The listing builds one solid part. Answer for the finished solid, in the listing's coordinates (mm). A direction names the side the tool comes from. Give positions to 0.01 mm unless a question says otherwise; leave off trailing zeros. Order: outer loops, then holes, each group sorted by start corner. A loop starts at its lowest first (then second) coordinate and runs counter-clockwise, first axis right, second up. Notation, with made-up numbers: (-8, -38.5) - (40, -38.5) arc R36 cw to (40, -3.5) - close; hole circle Ø11 at (58.25, -22.75). An arc over 180 degrees is marked (long way). Use a Markdown table: item, result. Add a question column.
1) Flat-ended cylindrical pins translate along their axes: pin 1 (10 mm diameter, centred on x = 62.5, y = 68, fed in from +Z); pin 2 (8 mm diameter, centred on y = 23, z = 55.5, fed in from -X); pin 3 (5 mm diameter, centred on x = 46.5, z = 36.5, fed in from -Y). Find the tip coordinate at first contact, or state that the pin passes through.
2) Find section B-B, the plane x = 10.5. Determine the outline of the cut face in (y, z), plus the area to 3 significant figures.
3) The mould has two halves that part along Z. Classify faces 1 (the face through (60.14, 45.69, 18.14)), 2 (the face through (112.2, 9.4, 97.8)), 3 (the face through (131.14, 46, 130)), 4 (the face through (55.832, 45.69, 138.224)): released by +Z, released by -Z, zero draft, split by the parting line, or undercut.
4) Straight lines are drawn through the part: line 1 (Z direction, x = 94, y = 11); line 2 (X direction, y = 18, z = 57); line 3 (Y direction, x = 22, z = 22.5). For each, find the intervals that lie inside material, in ascending order.
5) Find section C-C, the plane z = 133.5. Determine the outline of the cut face in (x, y).
6) Find section D-D, the plane y = 25.5. Determine the outline of the cut face in (x, z).
7) For faces 5 (the face through (70.85, 45.69, 18.66)), 6 (the face through (124.79, 9, 27)), 7 (the face through (6.35, 81, 128)), determine the directions among +Z, -Z, +X, -X, +Y, -Y from which every point of the face is accessible in a straight line to the end or side of a thin tool.
from build123d import *

# Parameters (mm, degrees)
F1_DEPTH = 45.0596
F2_DEPTH = 19.05


with BuildPart() as f1:
    # F0 (on Front) → F1 (new body)
    with BuildSketch(Plane.XZ):
        Polygon((0, 50.419), (0, 0), (54.864, 0), (65.5701, 36.8030026051), (76.2762, 0), (131.1402, 0), (131.1402, 50.419), (107.8484138495, 81.4324), (131.1402, 112.4458), (131.1402, 148.0566), (84.7852, 148.0566), (65.3923, 128.6637), (45.9994, 148.0566), (0, 148.0566), (0, 112.4458), (23.2917861505, 81.4324), align=None)
        Polygon((6.35, 114.5647761782), (6.35, 141.7066), (43.3691438789, 141.7066), (65.3923, 119.6834438789), (87.4154561211, 141.7066), (124.7902, 141.7066), (124.7902, 114.5647761782), (99.9070133581, 81.4324), (124.7902, 48.3000238218), (124.7902, 6.35), (81.0421936034, 6.35), (65.5701, 59.5364545624), (50.0980063966, 6.35), (6.35, 6.35), (6.35, 48.3000238218), (31.2331866419, 81.4324), align=None, mode=Mode.SUBTRACT)
        Polygon((43.3691438789, 141.7066), (6.35, 141.7066), (6.35, 114.5647761782), (31.2331866419, 81.4324), (6.35, 48.3000238218), (6.35, 6.35), (50.0980063966, 6.35), (65.5701, 59.5364545624), (81.0421936034, 6.35), (124.7902, 6.35), (124.7902, 48.3000238218), (99.9070133581, 81.4324), (124.7902, 114.5647761782), (124.7902, 141.7066), (87.4154561211, 141.7066), (65.3923, 119.6834438789), align=None)
    extrude(amount=-F1_DEPTH)

    # F0 (on Front) → F2 (cut, symmetric)
    with BuildSketch(Plane.XZ):
        Polygon((43.3691438789, 141.7066), (6.35, 141.7066), (6.35, 114.5647761782), (31.2331866419, 81.4324), (6.35, 48.3000238218), (6.35, 6.35), (50.0980063966, 6.35), (65.5701, 59.5364545624), (81.0421936034, 6.35), (124.7902, 6.35), (124.7902, 48.3000238218), (99.9070133581, 81.4324), (124.7902, 114.5647761782), (124.7902, 141.7066), (87.4154561211, 141.7066), (65.3923, 119.6834438789), align=None)
    extrude(amount=F2_DEPTH, both=True, mode=Mode.SUBTRACT)

    # F3: F1 across face


with BuildPart() as f1_1:
    add(f1.part)
    add(f1.part.mirror(Plane(origin=(65.5739873585, 45.0596, 73.343942561), x_dir=(1, 0, 0), z_dir=(0, 1, 0))))


solid = f1_1.part
The answers:
| question | item | result |
|---|---|---|
| 1 | pin 1 | z = 136.56 |
| 1 | pin 2 | x = 0.81 |
| 1 | pin 3 | y = 19.05 |
| 2 | outline | (0, 0) - (90.12, 0) - (90.12, 6.35) - (71.07, 6.35) - (71.07, 53.83) - (90.12, 53.83) - (90.12, 64.4) - (0, 64.4) - (0, 53.83) - (19.05, 53.83) - (19.05, 6.35) - (0, 6.35) - close; (0, 98.46) - (90.12, 98.46) - (90.12, 109.04) - (71.07, 109.04) - (71.07, 141.71) - (90.12, 141.71) - (90.12, 148.06) - (0, 148.06) - (0, 141.71) - (19.05, 141.71) - (19.05, 109.04) - (0, 109.04) - close |
| 2 | area | 7,220 mm2 |
| 3 | face 1 | released by -Z |
| 3 | face 2 | undercut |
| 3 | face 3 | zero draft |
| 3 | face 4 | released by +Z |
| 4 | line 1 | 0 to 6.35, 141.71 to 148.06 |
| 4 | line 2 | 4.94 to 12.88, 64.83 to 66.31, 118.26 to 126.2 |
| 4 | line 3 | 19.05 to 71.07 |
| 5 | outline | (0, 0) - (6.35, 0) - (6.35, 19.05) - (51.58, 19.05) - (51.58, 0) - (60.56, 0) - (60.56, 90.12) - (51.58, 90.12) - (51.58, 71.07) - (6.35, 71.07) - (6.35, 90.12) - (0, 90.12) - close; (70.23, 0) - (79.21, 0) - (79.21, 19.05) - (124.79, 19.05) - (124.79, 0) - (131.14, 0) - (131.14, 90.12) - (124.79, 90.12) - (124.79, 71.07) - (79.21, 71.07) - (79.21, 90.12) - (70.23, 90.12) - close |
| 6 | outline | (0, 0) - (54.86, 0) - (65.57, 36.8) - (76.28, 0) - (131.14, 0) - (131.14, 50.42) - (107.85, 81.43) - (131.14, 112.45) - (131.14, 148.06) - (84.79, 148.06) - (65.39, 128.66) - (46, 148.06) - (0, 148.06) - (0, 112.45) - (23.29, 81.43) - (0, 50.42) - close |
| 7 | face 5 | -Z, +Y, -Y |
| 7 | face 6 | -Y |
| 7 | face 7 | +Y |
